from build123d import *

# Parameters (mm, degrees)
SKETCH5_W            = 10
SKETCH5_H            = 30
BOSS_EXTRUDE5_DEPTH  = 3
M3_CLEARANCE_HOLE1_D = 3.6


with BuildPart() as part:
    # Sketch5 → Boss-Extrude5 (new body)
    with BuildSketch(Plane(origin=(0, 0, 0), x_dir=(1, 0, 0), z_dir=(0, 1, 0))):
        with Locations((-5, 51)):
            Rectangle(SKETCH5_W, SKETCH5_H)
        Polygon((0, 0), (34.5, 0), (34.5, 235.74), (0, 235.74), (0, 66), (0, 36), align=None)
        Polygon((69, 0), (69, 36), (69, 66), (69, 235.74), (34.5, 235.74), (34.5, 0), align=None)
        with Locations((74, 51)):
            Rectangle(SKETCH5_W, SKETCH5_H)
    extrude(amount=BOSS_EXTRUDE5_DEPTH)

    # M3 Clearance Hole1 (through all)
    with Locations(Plane(origin=(0, 3, 0), x_dir=(1, 0, 0), z_dir=(0, 1, 0))):
        with Locations((75.5, 50.420635549), (75.5, 42.420635549)):
            m3_clearance_hole1 = Hole(M3_CLEARANCE_HOLE1_D / 2)

    # Mirror1: M3 Clearance Hole1 across plane
    add(m3_clearance_hole1.mirror(Plane(origin=(34.5, 0, 0), x_dir=(0, 0, 1), z_dir=(1, 0, 0))), mode=Mode.SUBTRACT)


solid = part.part
Design review of the part built by this model. Coordinates are the model's own, in mm. Coordinates: 2 decimals unless noted, no trailing zeros. Order: outer loops, then holes, each group sorted by start corner. A loop starts at its lowest first (then second) coordinate and runs counter-clockwise, first axis right, second up.
Item 1: Take a section at A-A, the plane y = 2.2. Write out the cut boundary in (x, z), then the cut area to 3 significant figures.
Item 2: For line 1 (Z direction, x = -6.5, y = 0.8); line 2 (X direction, y = 1.3, z = -97), list the stretches that pass through material, from the lowest coordinate up.
Item 3: For pin 1 Ø0.9 at (x, y) = (-4, 2) entering from -Z; pin 2 Ø1.5 at (y, z) = (1, -14) entering from +X; pin 3 Ø0.9 at (x, y) = (-5.5, 1.5) entering from +Z, all flat-tipped, find the tip position at first contact; note any pin that passes through.
Item 4: Take a section at B-B, the plane z = -169.5. Write out the cut boundary in (x, y).
The answers:
1. outline: (-10, -66) - (0, -66) - (0, -235.74) - (69, -235.74) - (69, -66) - (79, -66) - (79, -36) - (69, -36) - (69, 0) - (0, 0) - (0, -36) - (-10, -36) - close; hole circle Ø3.6 at (-6.5, -50.42); hole circle Ø3.6 at (-6.5, -42.42); hole circle Ø3.6 at (75.5, -50.42); hole circle Ø3.6 at (75.5, -42.42)
1. area: 16,800 mm2
2. line 1: z = -66 to -52.22, -48.62 to -44.22, -40.62 to -36
2. line 2: x = 0 to 69
3. pin 1: stops at z = -66
3. pin 2: stops at x = 69
3. pin 3: stops at z = -36
4. outline: (0, 0) - (69, 0) - (69, 3) - (0, 3) - close
